```python
from build123d import *

# Parameters (mm, degrees)
SKETCH_1_W          = 1200
SKETCH_1_H          = 800
EXTRUDE_1_DEPTH     = 50
SKETCH_2_W          = 50
SKETCH_2_H          = 50
EXTRUDE_2_DEPTH     = 700
SKETCH_3_W          = 50
SKETCH_3_H          = 50
EXTRUDE_3_DEPTH     = 700
SKETCH_4_W          = 50
SKETCH_4_H          = 50
EXTRUDE_4_DEPTH     = 700
SKETCH_5_W          = 50
SKETCH_5_H          = 50
EXTRUDE_5_DEPTH     = 700
SKETCH_6_R          = 200
CUT_EXTRUDE_1_DEPTH = 20


with BuildPart() as part:
    # 草图1 → 凸台-拉伸1 (new body)
    with BuildSketch(Plane.XY):
        Rectangle(SKETCH_1_W, SKETCH_1_H)
    extrude(amount=EXTRUDE_1_DEPTH)

    # 草图2 → 凸台-拉伸2 (add)
    with BuildSketch(Plane.XY):
        with Locations((525, 350)):
            Rectangle(SKETCH_2_W, SKETCH_2_H)
    extrude(amount=EXTRUDE_2_DEPTH)

    # 草图3 → 凸台-拉伸3 (add)
    with BuildSketch(Plane.XY):
        with Locations((525, -350)):
            Rectangle(SKETCH_3_W, SKETCH_3_H)
    extrude(amount=EXTRUDE_3_DEPTH)

    # 草图4 → 凸台-拉伸4 (add)
    with BuildSketch(Plane.XY):
        with Locations((-525, 350)):
            Rectangle(SKETCH_4_W, SKETCH_4_H)
    extrude(amount=EXTRUDE_4_DEPTH)

    # 草图5 → 凸台-拉伸5 (add)
    with BuildSketch(Plane.XY):
        with Locations((-525, -350)):
            Rectangle(SKETCH_5_W, SKETCH_5_H)
    extrude(amount=EXTRUDE_5_DEPTH)

    # 草图6 → 切除-拉伸1 (cut)
    with BuildSketch(Plane.XY):
        Circle(SKETCH_6_R)
    extrude(amount=CUT_EXTRUDE_1_DEPTH, mode=Mode.SUBTRACT)


solid = part.part
```
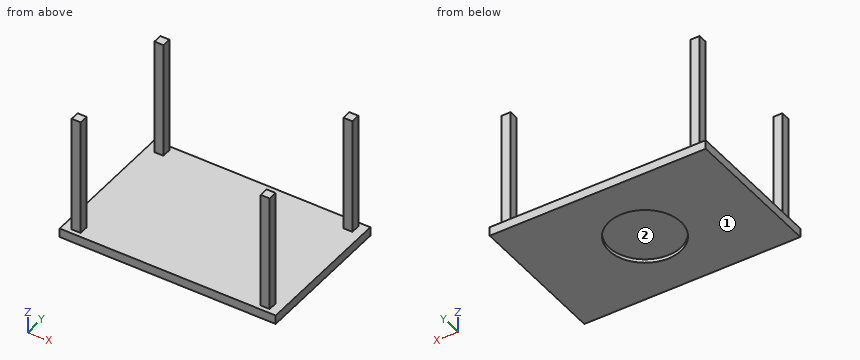
For this review, take the finished solid that the model builds, in its own axes (mm). Face numbers are marked on the shaded views. Round coordinates to 2 decimals unless told otherwise and drop trailing zeros. Order: outer loops, then holes, each group sorted by start corner. A loop starts at its lowest first (then second) coordinate and runs counter-clockwise, first axis right, second up. Notation, with made-up numbers: (6.25, 80.25) -> (46.25, 80.25) arc R9 cw to (46.25, 96.25) -> close; hole circle Ø5 at (48, 75). An arc over 180 degrees is marked (long way). Use a Markdown table: item, result.
Item 1: For pin 1 (15 mm diameter, centred on y = 342.5, z = 309.5, fed in from +X); pin 2 (15 mm diameter, centred on x = 535, z = 410, fed in from -Y); pin 3 (15 mm diameter, centred on y = -340, z = 455.5, fed in from -X), all flat-tipped, find the tip position at first contact; note any pin that passes through.
Resolved:
| item | result |
|---|---|
| pin 1 | stops at x = 550 |
| pin 2 | stops at y = -375 |
| pin 3 | stops at x = -550 |
Item 2: Take a section at D-D (x = -414.5). State the section outline as (y, z) points, plus the area to 3 significant figures.
Resolved:
| item | result |
|---|---|
| outline | (-400, 0) -> (400, 0) -> (400, 50) -> (-400, 50) -> close |
| area | 40,000 mm² |
Item 3: Take a section at C-C (y = 0). State the section outline as (x, z) points, plus the area to 3 significant figures.
Resolved:
| item | result |
|---|---|
| outline | (-600, 0) -> (-200, 0) -> (-200, 20) -> (200, 20) -> (200, 0) -> (600, 0) -> (600, 50) -> (-600, 50) -> close |
| area | 52,000 mm² |
Item 4: Take a section at B-B (x = 0). State the section outline as (y, z) points.
Resolved:
| item | result |
|---|---|
| outline | (-400, 0) -> (-200, 0) -> (-200, 20) -> (200, 20) -> (200, 0) -> (400, 0) -> (400, 50) -> (-400, 50) -> close |
Item 5: Draft analysis for pull direction X (two halves, no side actions). For the marked faces 1 and 2, state which applies: +X half, -X half, draft (parallel to the pull), parting line (faces both ways), or undercut.
Resolved:
| item | result |
|---|---|
| face 1 | draft |
| face 2 | undercut |
Item 6: Take a section at A-A (z = 419). State the section outline as (x, y) points, plus the area to 3 significant figures.
Resolved:
| item | result |
|---|---|
| outline | (-550, -375) -> (-500, -375) -> (-500, -325) -> (-550, -325) -> close; (-550, 325) -> (-500, 325) -> (-500, 375) -> (-550, 375) -> close; (500, -375) -> (550, -375) -> (550, -325) -> (500, -325) -> close; (500, 325) -> (550, 325) -> (550, 375) -> (500, 375) -> close |
| area | 10,000 mm² |
Item 7: For line 1 along Y through (x, z) = (0, 11.5); line 2 along Z through (x, y) = (53.5, 227.5); line 3 along Y through (x, z) = (540, 221), list the stretches that pass through material, from the lowest coordinate up. Write a range as [from, to].
Resolved:
| item | result |
|---|---|
| line 1 | y = [-400, -200], [200, 400] |
| line 2 | z = [0, 50] |
| line 3 | y = [-375, -325], [325, 375] |
